```python
from build123d import *

# Parameters (mm, degrees)
BOSS_EXTRUDE1_DEPTH = 4
SKETCH2_W           = 10
SKETCH2_H           = 1.5
BOSS_EXTRUDE3_DEPTH = 30


with BuildPart() as part:
    # Sketch1 → Boss-Extrude1 (new body)
    with BuildSketch(Plane(origin=(0, 0, 0), x_dir=(1, 0, 0), z_dir=(0, 1, 0))):
        with BuildLine():
            Line((32.5, -15), (32.5, 15))
            add(Edge.make_bspline(
                [(32.5, 15), (-18.815789474, 15), (-32.5, 4)],
                knots=[1.570796327, 1.570796327, 1.570796327, 2.871659858, 2.871659858, 2.871659858], degree=2, weights=[1, 0.795822426, 1]))
            Line((-32.5, 4), (-32.5, -4))
            add(Edge.make_bspline(
                [(-32.5, -4), (-18.815789474, -15), (32.5, -15)],
                knots=[3.411525449, 3.411525449, 3.411525449, 4.71238898, 4.71238898, 4.71238898], degree=2, weights=[1, 0.795822426, 1]))
        make_face()
    extrude(amount=BOSS_EXTRUDE1_DEPTH)

    # Sketch2 → Boss-Extrude3 (add)
    with BuildSketch(Plane(origin=(0, 4, 0), x_dir=(1, 0, 0), z_dir=(0, 1, 0))):
        with Locations((-27.5, -1.25)):
            Rectangle(SKETCH2_W, SKETCH2_H)
        with Locations((-27.5, 1.25)):
            Rectangle(SKETCH2_W, SKETCH2_H)
    extrude(amount=BOSS_EXTRUDE3_DEPTH)


solid = part.part
```
Could you check a few things on this model? Use its own coordinates, in mm. A direction names the side the tool comes from. Give positions to 0.01 mm unless a question says otherwise; leave off trailing zeros. Loops run counter-clockwise (first coordinate to the right, second up) from the corner with the lowest first, then second, coordinate; pieces in that order, holes last. Notation, with made-up numbers: (4.5, 69.25) - (47.5, 69.25) arc R18 cw to (47.5, 80.25) - close; hole circle Ø9 at (6.25, 56.25). An arc over 180 degrees is marked (long way). Use one line per item in the form item = value.
1. On a 3-axis mill with a long thin cutter (end or side, diameter ignored), from which of +Z, -Z, +X, -X, +Y, -Y can I reach the whole of each face in a straight line? I mean faces 4 (the face through (-28, 34, 1)), 5 (the face through (-22.5, 19, -1)), 6 (the face through (-28, 19, -2)), 7 (the face through (-32.5, 17, -1)), 8 (the face through (-28, 19, 0.5)). Say none if no direction works.
Response values:
face_4 = +Z, -Z, +X, -X, +Y
face_5 = +Z, -Z, +X, +Y
face_6 = -Z, +X, -X, +Y
face_7 = +Z, -Z, -X, +Y, -Y
face_8 = +X, -X, +Y
2. I want a section at B-B (z = -3). Please give me the cut outline in (x, y).
Response values:
outline = (-32.5, 0) - (32.5, 0) - (32.5, 4) - (-32.5, 4) - close
3. I need wall thicknesses on probe 1 along Z at (x, y) = (-27.5, 4.5); probe 2 along Y at (x, z) = (29.5, -6); probe 3 along X at (y, z) = (10.5, -1.5). Which ranges of each line are inside material? Lowest first, please.
Response values:
probe_1 = -2 to -0.5, 0.5 to 2
probe_2 = 0 to 4
probe_3 = -32.5 to -22.5
4. I'm going to push flat-ended pins straight in: pin 1 Ø1.6 at (y, z) = (24.5, 1) entering from +X; pin 2 Ø3 at (x, z) = (23.5, 1.5) entering from +Y; pin 3 Ø10 at (x, y) = (0, 10) entering from +Z; pin 4 Ø4 at (x, y) = (-25.5, 18.5) entering from +Z. Where does each tip first touch, or does it pass through?
Response values:
pin_1 = -22.5
pin_2 = 4
pin_3 = through
pin_4 = 2
5. Thinking about a two-plate mould opening in Z: for faces 1 (the face through (-28, 19, -0.5)), 2 (the face through (-28, 19, 2)), 3 (the face through (-22.5, 19, 1)), which applies, released by +Z, released by -Z, zero draft, split by the parting line, or undercut?
Response values:
face_1 = undercut
face_2 = released by +Z
face_3 = zero draft
6. I want a section at A-A (y = 22). Please give me the cut outline in (x, z), and give its area (3 significant figures).
Response values:
outline = (-32.5, -2) - (-22.5, -2) - (-22.5, -0.5) - (-32.5, -0.5) - close; (-32.5, 0.5) - (-22.5, 0.5) - (-22.5, 2) - (-32.5, 2) - close
area = 30.0 mm²
